Can you work these out from the model? Positions are in its coordinate system, mm. A direction names the side the tool comes from. Coordinates: 2 decimals unless noted, no trailing zeros. Loops run counter-clockwise (first coordinate to the right, second up) from the corner with the lowest first, then second, coordinate; pieces in that order, holes last.
```python
from build123d import *

# Parameters (mm, degrees)
F0_R     = 25.4
F0_R_2   = 12.5
F1_DEPTH = 6
F3_DEPTH = 2
F4_R     = 3.175
F5_DEPTH = 6.001


with BuildPart() as f1:
    # F0 (on Front) → F1 (new body)
    with BuildSketch(Plane.XZ):
        Circle(F0_R)
        Circle(F0_R_2, mode=Mode.SUBTRACT)
    extrude(amount=F1_DEPTH)

    # F2 (on face) → F3 (cut)
    with BuildSketch(Plane.XZ.offset(6)):
        with BuildLine():
            ThreePointArc((-6.35, -24.5934442484), (0, -25.4), (6.35, -24.5934442484))
            Line((6.35, -24.5934442484), (6.35, -10.7669633602))
            ThreePointArc((6.35, -10.7669633602), (0, -12.5), (-6.35, -10.7669633602))
            Line((-6.35, -10.7669633602), (-6.35, -24.5934442484))
        make_face()
    extrude(amount=-F3_DEPTH, mode=Mode.SUBTRACT)

    # F4 (on face) → F5 (cut, through all)
    with BuildSketch(Plane.XZ.offset(6)):
        with Locations((-19.05, 0)):
            Circle(F4_R)
    extrude(amount=-F5_DEPTH, mode=Mode.SUBTRACT)


solid = f1.part
```
(1) Which directions (+Z, -Z, +X, -X, +Y, -Y) give clear straight access to the entire face, cutting with the end or side of a thin tool? Please do faces 5 (the flat face through (0, -4, -18)), 6 (the flat face through (5, -6, 12)).
Check values:
face 5: -Z, -Y
face 6: +Z, -Z, +X, -X, -Y
(2) I want a section at A-A on z = 0. Write out the boundary of the cut face in (x, y) (3 decimals), then the cut area to 3 significant figures.
Check values:
outline: (-25.4, -6) - (-22.225, -6) - (-22.225, 0) - (-25.4, 0) - close; (-15.875, -6) - (-12.5, -6) - (-12.5, 0) - (-15.875, 0) - close; (12.5, -6) - (25.4, -6) - (25.4, 0) - (12.5, 0) - close
area: 117 mm2
(3) I'm going to push flat-ended pins straight in: pin 1 (4 mm diameter, centred on x = 0.5, z = -18, fed in from -Y); pin 2 (1.6 mm diameter, centred on y = -4.5, z = -17, fed in from -X); pin 3 (1 mm diameter, centred on x = -2, y = -2.5, fed in from -Z). Where does each tip first touch, or does it pass through?
Check values:
pin 1: stops at y = -4
pin 2: stops at x = -19.56
pin 3: stops at z = -25.36
(4) I want a section at B-B on x = 0. Write out the boundary of the cut face in (y, z).
Check values:
outline: (-6, 12.5) - (0, 12.5) - (0, 25.4) - (-6, 25.4) - close; (-4, -25.4) - (0, -25.4) - (0, -12.5) - (-4, -12.5) - close
(5) If I drill on probe 1 along Z at (x, y) = (-21, -2.7); probe 2 along Z at (x, y) = (-17.5, -1.8); probe 3 along X at (y, z) = (-3.8, 7), over which ranges is the centre line in solid material (lowest first)?
Check values:
probe 1: z = -14.29 to -2.51, 2.51 to 14.29
probe 2: z = -18.41 to -2.77, 2.77 to 18.41
probe 3: x = -24.42 to -10.36, 10.36 to 24.42
(6) If we mould it in two halves opening along X, with no side actions, what happens to faces 1 (the flat face through (-6.35, -5, -18)), 2 (the cylindrical face through (-3.307, -2.958, 25.184)), 3 (the flat face through (5, 0, 12)), 4 (the cylindrical face through (-16.02, -3.04, 0.95))? For each: released by +X, released by -X, zero draft, split by the parting line, or undercut.
Check values:
face 1: undercut
face 2: split by the parting line
face 3: zero draft
face 4: undercut
(7) I want a section at D-D on y = -5. Write out the boundary of the cut face in (x, z) (3 decimals), then the cut area to 3 significant figures.
Check values:
outline: (-6.35, -24.593) - (-6.35, -10.767) arc R12.5 cw (long way) to (6.35, -10.767) - (6.35, -24.593) arc R25.4 ccw (long way) to start; hole circle Ø6.35 at (-19.05, 0)
area: 1,340 mm2
(8) I want a section at C-C on y = -1.45. Write out the boundary of the cut face in (x, z) (3 decimals), then the cut area to 3 significant figures.
Check values:
outline: circle Ø50.8 at (0, 0); hole circle Ø6.35 at (-19.05, 0); hole circle Ø25 at (0, 0)
area: 1,500 mm2
